Autodesk Inventor part; units mm, degrees
ref_plane "YZ Plane" through (0, 0, 0) normal (1, 0, 0) x (0, 1, 0)
ref_plane "XZ Plane" through (0, 0, 0) normal (0, 1, 0) x (-1, 0, 0)
ref_plane "XY Plane" through (0, 0, 0) normal (0, 0, 1) x (1, 0, 0)
sketch "Sketch1" plane through (0, 0, 0) normal (0, 0, 1) x (1, 0, 0)
  circle A0 centre (0, 0) radius 7.5
  circle A1 centre (0, 0) radius 10
  dimension "d0" = 15
  dimension "d1" = 20
extrude "Extrusion1" add sketch "Sketch1" along normal blind 24
sketch "Sketch2" plane through (0, 0, 0) normal (0, 0, -1) x (-1, 0, 0)
  circle A0 centre (0, 0) radius 7
  circle A1 centre (0, 0) radius 7.5
  circle A2 centre (0, 0) radius 10
  circle A3 centre (0, 0) radius 7.5
  circle A4 centre (0, 0) radius 10
  circle A5 centre (0, 0) radius 7.5
  circle A6 centre (0, 0) radius 10
  circle A7 centre (0, 0) radius 7.5
  dimension "d4" = 14
extrude "Extrusion2" add sketch "Sketch2" along normal blind 150 contours A1 | A2
sketch "Sketch3" plane through (0, 0, 24) normal (0, 0, 1) x (1, 0, 0)
  circle A0 centre (0, 0) radius 10
  circle A1 centre (0, 0) radius 7.5
  circle A2 centre (0, 0) radius 8
  dimension "d7" = 0.5
extrude "Extrusion3" add sketch "Sketch3" along normal blind 1 contours A0
sketch "Sketch4" plane through (0, 0, 25) normal (0, 0, 1) x (1, 0, 0)
  circle A0 centre (0, 0) radius 10
  circle A1 centre (0, 0) radius 7.5
extrude "Extrusion4" add sketch "Sketch4" along normal blind 3
sketch "Sketch5" plane through (0, 0, -150) normal (0, 0, -1) x (-1, 0, 0)
  line L0 (-12.5, -10) -> (12.5, -10)
  circle A0 centre (0, 0) radius 10
  line L1 (-12.5, -10) -> (-12.5, 12)
  line L2 (-12.5, 12) -> (12.5, 12)
  line L3 (12.5, 12) -> (12.5, -10)
  circle A1 centre (-7.62, 7.24) radius 1.27
  circle A2 centre (7.62, 7.24) radius 1.27
  line L4 (-7.62, 7.24) -> (7.62, 7.24) construction
  point P0 (0, 7.24)
  point P1 (0, -10)
  point P2 (0, -10)
  point P3 (-7.9828, 6.0229)
  point P4 (-6.423, 7.6645)
  point P5 (6.423, 7.6645)
  point P6 (7.9828, 6.0229)
  dimension "d12" = 25
  dimension "d13" = 22
  dimension "d14" = 15.24
  dimension "d15" = 17.24
  dimension "d16" = 2.54
extrude "Extrusion5" add sketch "Sketch5" against normal blind 3
extrude "Extrusion6" cut sketch "Sketch5" against normal blind 3 contours A1 A0 | A0 A1 | A2 A0 | A0 A2
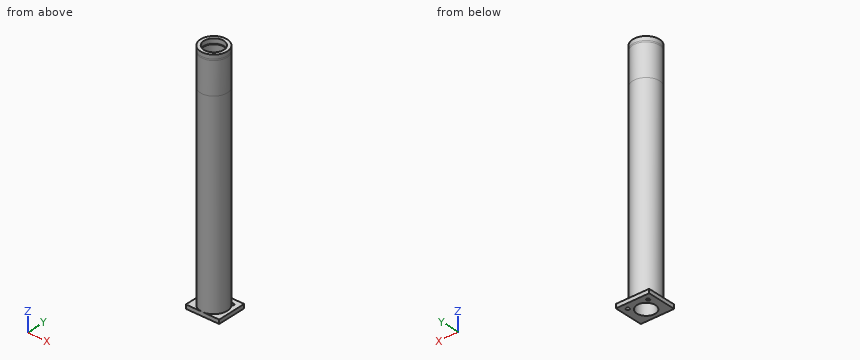
Geometry: final body of the model. Coordinates: model frame, mm. Coordinates: 2 decimals unless noted, no trailing zeros. Order: outer loops, then holes, each group sorted by start corner. A loop starts at its lowest first (then second) coordinate and runs counter-clockwise, first axis right, second up. Notation, with made-up numbers: M -39.5,-0.5 L -31.5,-0.5 A27 ccw -31.5,17.5 Z; hole C 66,84 d1. An arc over 180 degrees is marked long. Answer as CSV lines item,"result".
Q1. First-contact query: P1, Ø1.5, axis at y = 6.5, z = -108, coming from the -X side; P2, Ø10, axis at x = -7.5, z = 3.5, coming from the +Y side; P3, Ø0.5, axis at x = 7.5, y = 6.5, coming from the -Z side. Flat tips, straight axial feed; report the tip coordinate or a pass-through.
Answers:
P1,"stops at x = -8.18"
P2,"stops at y = 9.68"
P3,"stops at z = -147"
Q2. Section C-C on z = -38.5. Return the cut outline in (x, y).
Answers:
outline,"C 0,0 d20; hole C 0,0 d14"
Q3. Section D-D on z = 10. Return the cut outline in (x, y).
Answers:
outline,"C 0,0 d20; hole C 0,0 d15"
Q4. Line query: probe 1 along X at (y, z) = (7.24, -148.3); probe 2 along Y at (x, z) = (0, 8); probe 3 along X at (y, z) = (-0.5, -130). Output: solid intervals per line, ascending. Write a range as [from, to].
Answers:
probe 1,"x = [-12.5, -8.89], [-6.35, 6.35], [8.89, 12.5]"
probe 2,"y = [-10, -7.5], [7.5, 10]"
probe 3,"x = [-9.99, -6.98], [6.98, 9.99]"
Q5. Section A-A on y = 0. Return the cut outline in (x, z).
Answers:
outline,"M -12.5,-150 L -7,-150 L -7,0 L -7.5,0 L -7.5,24 L -8,24 L -8,25 L -7.5,25 L -7.5,28 L -10,28 L -10,-147 L -12.5,-147 Z; M 7,-150 L 12.5,-150 L 12.5,-147 L 10,-147 L 10,28 L 7.5,28 L 7.5,25 L 8,25 L 8,24 L 7.5,24 L 7.5,0 L 7,0 Z"
Q6. Section B-B on x = 1.5. Return the cut outline in (y, z), and give its area (3 significant figures).
Answers:
outline,"M -10,-150 L -6.84,-150 L -6.84,0 L -7.35,0 L -7.35,24 L -7.86,24 L -7.86,25 L -7.35,25 L -7.35,28 L -9.89,28 L -9.89,-147 L -10,-147 Z; M 6.84,-150 L 12,-150 L 12,-147 L 9.89,-147 L 9.89,28 L 7.35,28 L 7.35,25 L 7.86,25 L 7.86,24 L 7.35,24 L 7.35,0 L 6.84,0 Z"
area,"1,060 mm^2"
